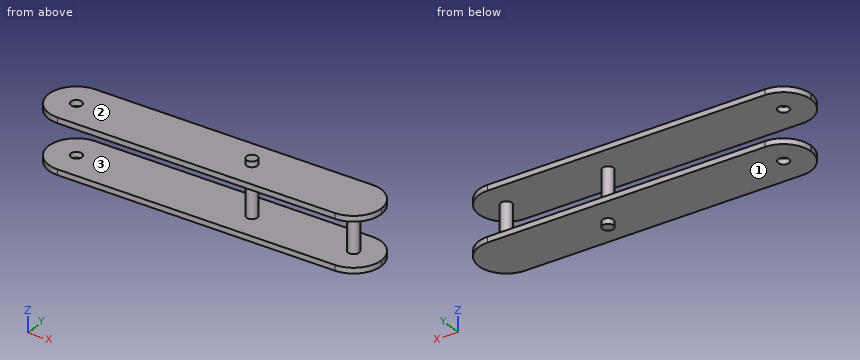
from build123d import *

# Parameters (mm, degrees)
CROQUIS2_R              = 3
SALIENTE_EXTRUIR1_DEPTH = 18
CROQUIS3_R              = 3
SALIENTE_EXTRUIR2_DEPTH = 18
CROQUIS4_W              = 3
CROQUIS4_H              = 30
SALIENTE_EXTRUIR3_DEPTH = 110
CROQUIS5_W              = 3
CROQUIS5_H              = 30
SALIENTE_EXTRUIR4_DEPTH = 70
CORTAR_EXTRUIR1_DEPTH   = 70
CORTAR_EXTRUIR2_DEPTH   = 70
CROQUIS8_R              = 3
CORTAR_EXTRUIR3_DEPTH   = 70
CROQUIS9_R              = 3
SALIENTE_EXTRUIR6_DEPTH = 30


with BuildPart() as part:
    # Croquis2 → Saliente-Extruir1 (new body)
    with BuildSketch(Plane.XY):
        Circle(CROQUIS2_R)
    extrude(amount=SALIENTE_EXTRUIR1_DEPTH)

    # Croquis3 → Saliente-Extruir2 (add)
    with BuildSketch(Plane.XY):
        Circle(CROQUIS3_R)
    extrude(amount=-SALIENTE_EXTRUIR2_DEPTH)

    # Croquis4 → Saliente-Extruir3 (add)
    with BuildSketch(Plane(origin=(0, 0, 0), x_dir=(0, 0, -1), z_dir=(1, 0, 0))):
        with Locations((-13.5, 0)):
            Rectangle(CROQUIS4_W, CROQUIS4_H)
        with Locations((13.5, 0)):
            Rectangle(CROQUIS4_W, CROQUIS4_H)
    extrude(amount=-SALIENTE_EXTRUIR3_DEPTH)

    # Croquis5 → Saliente-Extruir4 (add)
    with BuildSketch(Plane(origin=(0, 0, 0), x_dir=(0, 0, -1), z_dir=(1, 0, 0))):
        with Locations((-13.5, 0)):
            Rectangle(CROQUIS5_W, CROQUIS5_H)
        with Locations((13.5, 0)):
            Rectangle(CROQUIS5_W, CROQUIS5_H)
    extrude(amount=SALIENTE_EXTRUIR4_DEPTH)

    # Croquis6 → Cortar-Extruir1 (cut)
    with BuildSketch(Plane.XY.offset(15)):
        with BuildLine():
            Line((-110, -0.185040896), (-110, -15))
            Line((-110, -15), (-95.185040896, -15))
            ThreePointArc((-95.185040896, -15), (-105.607408735, -10.607408735), (-110, -0.185040896))
        make_face()
        with BuildLine():
            Line((-110, 15), (-110, 0.185040896))
            ThreePointArc((-110, 0.185040896), (-105.607408735, 10.607408735), (-95.185040896, 15))
            Line((-95.185040896, 15), (-110, 15))
        make_face()
    extrude(amount=-CORTAR_EXTRUIR1_DEPTH, mode=Mode.SUBTRACT)

    # Croquis7 → Cortar-Extruir2 (cut)
    with BuildSketch(Plane.XY.offset(15)):
        with BuildLine():
            ThreePointArc((55, 15), (65.606601718, 10.606601718), (70, 0))
            Line((70, 0), (70, 15))
            Line((70, 15), (55, 15))
        make_face()
        with BuildLine():
            ThreePointArc((70, 0), (65.606601718, -10.606601718), (55, -15))
            Line((55, -15), (70, -15))
            Line((70, -15), (70, 0))
        make_face()
    extrude(amount=-CORTAR_EXTRUIR2_DEPTH, mode=Mode.SUBTRACT)

    # Croquis8 → Cortar-Extruir3 (cut)
    with BuildSketch(Plane.XY.offset(15)):
        with Locations((-95, 0)):
            Circle(CROQUIS8_R)
    extrude(amount=-CORTAR_EXTRUIR3_DEPTH, mode=Mode.SUBTRACT)

    # Croquis9 → Saliente-Extruir6 (add)
    with BuildSketch(Plane.XY.offset(15)):
        with Locations((55, 0)):
            Circle(CROQUIS9_R)
    extrude(amount=-SALIENTE_EXTRUIR6_DEPTH)


solid = part.part
Geometry check sheet. Reference: the model listing, model coordinates, mm. Face numbers are marked on the shaded views. Round coordinates to 2 decimals unless told otherwise and drop trailing zeros. Order: outer loops, then holes, each group sorted by start corner. A loop starts at its lowest first (then second) coordinate and runs counter-clockwise, first axis right, second up. Notation, with made-up numbers: M 29,-35 L 85,-35 A22 ccw 85,-19 Z; hole C 6.5,54 d7. An arc over 180 degrees is marked long. Answer in a Markdown table with one row per item. Add a question column.
Item 1: Sectioned sample at D-D, the plane z = -9.5. Enter the section's corners in (x, y), plus the area to 3 significant figures.
Item 2: Sectioned sample at C-C, the plane x = 0. Enter the section's corners in (y, z).
Item 3: Depth check by flat-ended pin: pin 1 Ø10 at (x, z) = (-19.5, -3.5) entering from +Y; pin 2 Ø8 at (x, y) = (-95, 0) entering from -Z; pin 3 Ø10 at (y, z) = (-8, 14.5) entering from -X; pin 4 Ø12 at (x, y) = (-21, 1.5) entering from +Z. Enter the tip coordinate at first touch or a pass-through.
Item 4: Sectioned sample at B-B, the plane y = 13.5. Enter the section's corners in (x, z), plus the area to 3 significant figures.
Item 5: Sectioned sample at A-A, the plane x = 32. Enter the section's corners in (y, z), plus the area to 3 significant figures.
Item 6: Material ranges on L1, parallel to Z at x = 12, y = -8.5; L2, parallel to Y at x = -95, z = 13.2; L3, parallel to X at y = -0.5, z = -2.5, recorded low to high. Write a range as [from, to].
Item 7: Draft check along Z on the marked faces 1, 2 and 3. Enter one of: released by +Z, released by -Z, zero draft, split by the parting line, or undercut.
Filled in:
| question | item | result |
|---|---|---|
| 1 | outline | C 0,0 d6; C 55,0 d6 |
| 1 | area | 56.5 mm² |
| 2 | outline | M -15,-15 L -3,-15 L -3,-18 L 3,-18 L 3,-15 L 15,-15 L 15,-12 L 3,-12 L 3,12 L 15,12 L 15,15 L 3,15 L 3,18 L -3,18 L -3,15 L -15,15 L -15,12 L -3,12 L -3,-12 L -15,-12 Z |
| 3 | pin 1 | passes through |
| 3 | pin 2 | stops at z = -15 |
| 3 | pin 3 | stops at x = -109.7 |
| 3 | pin 4 | stops at z = 15 |
| 4 | outline | M -101.54,-15 L 61.54,-15 L 61.54,-12 L -101.54,-12 Z; M -101.54,12 L 61.54,12 L 61.54,15 L -101.54,15 Z |
| 4 | area | 978 mm² |
| 5 | outline | M -15,-15 L 15,-15 L 15,-12 L -15,-12 Z; M -15,12 L 15,12 L 15,15 L -15,15 Z |
| 5 | area | 180 mm² |
| 6 | L1 | z = [-15, -12], [12, 15] |
| 6 | L2 | y = [-15, -3], [3, 15] |
| 6 | L3 | x = [-2.96, 2.96], [52.04, 57.96] |
| 7 | face 1 | released by -Z |
| 7 | face 2 | released by +Z |
| 7 | face 3 | undercut |
